```python
from build123d import *

# Parameters (mm, degrees)
F1_DEPTH = 850
F2_W     = 40
F2_H     = 70
F3_DEPTH = 5
F4_R     = 5
F5_DEPTH = 25
F7_DEPTH = 150


with BuildPart() as f1:
    # F0 (on Top) → F1 (new body)
    with BuildSketch(Plane.XY):
        with BuildLine():
            Line((49.398924, -4.319251), (39.398924, -4.319251))
            ThreePointArc((39.398924, -4.319251), (28.691348, -47.741817), (24.398924, -92.258629))
            Line((24.398924, -92.258629), (24.398924, -106.582679))
            Line((24.398924, -106.582679), (24.398924, -144.319251))
            Line((24.398924, -144.319251), (64.398924, -144.319251))
            Line((64.398924, -144.319251), (64.398924, -106.582679))
            Line((64.398924, -106.582679), (64.398924, -92.258629))
            ThreePointArc((64.398924, -92.258629), (60.1065, -47.741817), (49.398924, -4.319251))
        make_face()
    extrude(amount=F1_DEPTH)

    # F2 (on face) → F3 (cut)
    with BuildSketch(Plane.XZ.offset(144.319251)):
        with Locations((44.398924, 185)):
            Rectangle(F2_W, F2_H)
    extrude(amount=-F3_DEPTH, mode=Mode.SUBTRACT)

    # F4 (on face) → F5 (cut)
    with BuildSketch(Plane.XZ.offset(139.319251)):
        with Locations((44.398924, 185)):
            Circle(F4_R)
    extrude(amount=-F5_DEPTH, mode=Mode.SUBTRACT)

    # F6 (on Right) → F7 (cut)
    with BuildSketch(Plane.YZ):
        with BuildLine():
            Line((-144.319251, 0), (-34.319251, 0))
            ThreePointArc((-34.319251, 0), (-84.06201, 36.565931), (-144.319251, 50))
            Line((-144.319251, 50), (-144.319251, 0))
        make_face()
    extrude(amount=F7_DEPTH, mode=Mode.SUBTRACT)


solid = f1.part
```
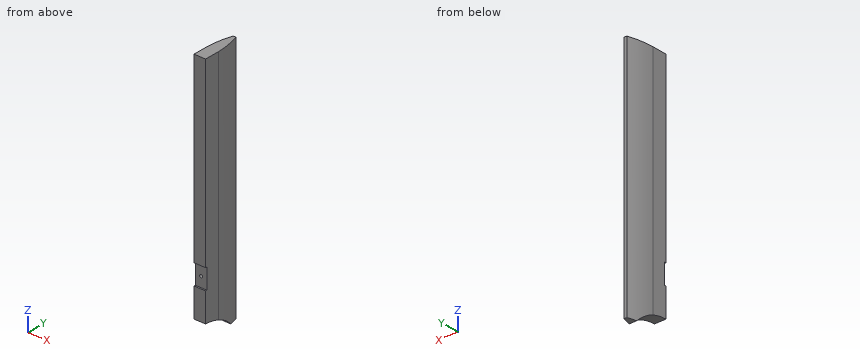
Model file for the job. Use its own axes, mm. Round coordinates to 2 decimals unless told otherwise and drop trailing zeros. Write each loop counter-clockwise with the first axis right and the second up, starting at its lowest first coordinate (ties: lowest second). Pieces come first, ordered by that corner, then holes. Notation, with made-up numbers: M -34,2 L -8,2 A28 cw -8,24 Z; hole C 33,-27.75 d7. An arc over 180 degrees is marked long. Put each result on its own line as item: value.
Item 1: Probe L1, parallel to Z at x = 58.5, y = -131; L2, parallel to Y at x = 45, z = 150.5; L3, parallel to X at y = -89.5, z = 604.5. List the from-to ranges inside material, lowest first. Write a range as from..to.
Responses:
L1: 49.25..850
L2: -139.32..-4.32
L3: 24.48..64.32
Item 2: Flat gauge pins, fed straight in: P1, Ø8, axis at x = 49.5, z = 397, coming from the +Y side; P2, Ø4, axis at x = 48, y = -143, coming from the -Z side; P3, Ø8, axis at x = 57, y = -61, coming from the -Z side; P4, Ø10, axis at x = 55.5, y = -108, coming from the -Z side. Where does each tip first touch, or does it go through?
Responses:
P1: y = -4.32
P2: z = 49.92
P3: z = 20.66
P4: z = 43.68
Item 3: Cut at B-B (y = -51.5). List the corners of the cut face in (x, z), and give its area (3 significant figures).
Responses:
outline: M 28.07,16.39 L 60.72,16.39 L 60.72,850 L 28.07,850 Z
area: 27,200 mm²
Item 4: Cut at A-A (z = 445). List the corners of the cut face in (x, y) (3 decimals), and give its area (3 significant figures).
Responses:
outline: M 24.399,-144.319 L 64.399,-144.319 L 64.399,-92.259 A307.35 ccw 49.399,-4.319 L 39.399,-4.319 A307.35 ccw 24.399,-92.259 Z
area: 4,670 mm²
